```python
from build123d import *

# Parameters (mm, degrees)
SKETCH1_R             = 150.5
BOSS_EXTRUDE1_DEPTH   = 6.35
SKETCH3_R             = 2.6
CUT_EXTRUDE2_DEPTH    = 10
M5X0_8_TAPPED_HOLE1_D = 4.2
CUT_EXTRUDE3_DEPTH    = 10


with BuildPart() as part:
    # Sketch1 → Boss-Extrude1 (new body)
    with BuildSketch(Plane(origin=(-388.281715987, 0, -288.185661777), x_dir=(1, 0, 0), z_dir=(0, 1, 0))):
        Polygon((1747.570833697, -13084.824581071), (1672.514355591, -13084.824581071), (1454.703489965, -13462.084066777), (1492.231729019, -13527.084883536), (1927.853460271, -13527.084883536), (1965.381699324, -13462.084066777), align=None)
        with Locations(Location((1710.042594644, -13357.997843795, 0), (0, 0, 270))):
            Circle(SKETCH1_R, mode=Mode.SUBTRACT)
        with BuildLine():
            Line((1730.692592416, -13114.874577827), (1730.692592416, -13095.074579966))
            ThreePointArc((1730.692592416, -13095.074579966), (1730.472922526, -13094.544249938), (1729.942592497, -13094.324580043))
            Line((1729.942592497, -13094.324580043), (1690.142596792, -13094.324580043))
            ThreePointArc((1690.142596792, -13094.324580043), (1689.612266761, -13094.544249935), (1689.392596873, -13095.074579966))
            Line((1689.392596873, -13095.074579966), (1689.392596873, -13114.874577827))
            ThreePointArc((1689.392596873, -13114.874577827), (1689.612266763, -13115.404907856), (1690.142596792, -13115.62457775))
            Line((1690.142596792, -13115.62457775), (1729.942592497, -13115.62457775))
            ThreePointArc((1729.942592497, -13115.62457775), (1730.472922528, -13115.404907859), (1730.692592416, -13114.874577827))
        make_face(mode=Mode.SUBTRACT)
        with BuildLine():
            Line((1492.669367808, -13507.342898369), (1509.816668952, -13497.442899438))
            ThreePointArc((1509.816668952, -13497.442899438), (1510.166113284, -13496.987494718), (1510.091187977, -13496.418380495))
            Line((1510.091187977, -13496.418380495), (1490.191190123, -13461.950573141))
            ThreePointArc((1490.191190123, -13461.950573141), (1489.735785404, -13461.60112881), (1489.166671181, -13461.676054117))
            Line((1489.166671181, -13461.676054117), (1472.019370034, -13471.57605305))
            ThreePointArc((1472.019370034, -13471.57605305), (1471.669925699, -13472.031457773), (1471.744851013, -13472.600571998))
            Line((1471.744851013, -13472.600571998), (1491.644848864, -13507.068379347))
            ThreePointArc((1491.644848864, -13507.068379347), (1492.100253585, -13507.41782368), (1492.669367808, -13507.342898369))
        make_face(mode=Mode.SUBTRACT)
        with BuildLine():
            Line((1948.065819252, -13471.576053055), (1930.918518105, -13461.676054122))
            ThreePointArc((1930.918518105, -13461.676054122), (1930.349403886, -13461.601128813), (1929.893999164, -13461.95057314))
            Line((1929.893999164, -13461.95057314), (1909.99400131, -13496.418380494))
            ThreePointArc((1909.99400131, -13496.418380494), (1909.919076, -13496.98749472), (1910.268520339, -13497.442899434))
            Line((1910.268520339, -13497.442899434), (1927.415821483, -13507.342898365))
            ThreePointArc((1927.415821483, -13507.342898365), (1927.984935702, -13507.417823673), (1928.440340423, -13507.068379346))
            Line((1928.440340423, -13507.068379346), (1948.340338275, -13472.600571997))
            ThreePointArc((1948.340338275, -13472.600571997), (1948.415263583, -13472.031457775), (1948.065819252, -13471.576053055))
        make_face(mode=Mode.SUBTRACT)
    extrude(amount=BOSS_EXTRUDE1_DEPTH)

    # Sketch3 → Cut-Extrude2 (cut)
    with BuildSketch(Plane(origin=(0, 6.35, 0), x_dir=(1, 0, 0), z_dir=(0, 1, 0))):
        with Locations(Location((1183.987460829, -12990.268662147, 0), (0, 0, 270))):
            Circle(SKETCH3_R)
        with Locations(Location((1146.487460829, -13055.220567431, 0), (0, 0, 270))):
            Circle(SKETCH3_R)
        with Locations(Location((1108.987460829, -13120.172472715, 0), (0, 0, 270))):
            Circle(SKETCH3_R)
        with Locations(Location((1221.487460829, -12925.316756863, 0), (0, 0, 270))):
            Circle(SKETCH3_R)
        with Locations(Location((1258.987460829, -12860.364851579, 0), (0, 0, 270))):
            Circle(SKETCH3_R)
        with Locations(Location((1459.534296487, -12990.268662148, 0), (0, 0, 270))):
            Circle(SKETCH3_R)
        with Locations(Location((1497.034296487, -13055.220567432, 0), (0, 0, 270))):
            Circle(SKETCH3_R)
        with Locations(Location((1534.534296487, -13120.172472716, 0), (0, 0, 270))):
            Circle(SKETCH3_R)
        with Locations(Location((1422.034296487, -12925.316756864, 0), (0, 0, 270))):
            Circle(SKETCH3_R)
        with Locations(Location((1384.534296487, -12860.364851581, 0), (0, 0, 270))):
            Circle(SKETCH3_R)
        with Locations(Location((1321.760878657, -13228.899221759, 0), (0, 0, 270))):
            Circle(SKETCH3_R)
        with Locations(Location((1246.760878657, -13228.899221759, 0), (0, 0, 270))):
            Circle(SKETCH3_R)
        with Locations(Location((1171.760878657, -13228.899221759, 0), (0, 0, 270))):
            Circle(SKETCH3_R)
        with Locations(Location((1396.760878657, -13228.899221759, 0), (0, 0, 270))):
            Circle(SKETCH3_R)
        with Locations(Location((1471.760878657, -13228.899221759, 0), (0, 0, 270))):
            Circle(SKETCH3_R)
    extrude(amount=-CUT_EXTRUDE2_DEPTH, mode=Mode.SUBTRACT)

    # M5x0.8 Tapped Hole1 (through all)
    with Locations(Plane(origin=(0, 6.35, 0), x_dir=(1, 0, 0), z_dir=(0, 1, 0))):
        with Locations((1321.760878658, -12912.312182018), (1321.760878658, -13069.812182018), (1382.033519255, -12924.301155648), (1261.48823806, -12924.301155648), (1185.361877562, -13148.562182018), (1165.608312991, -13090.370057293), (1225.880953589, -13194.765333114), (1417.640803726, -13194.765333114), (1458.159879754, -13148.562182018), (1477.913444324, -13090.370057293)):
            Hole(M5X0_8_TAPPED_HOLE1_D / 2)

    # Sketch9 → Cut-Extrude3 (cut)
    with BuildSketch(Plane(origin=(0, 6.35, 0), x_dir=(1, 0, 0), z_dir=(0, 1, 0))):
        with BuildLine():
            Line((1522.758854804, -13174.820007204), (1515.224433791, -13170.470007204))
            ThreePointArc((1515.224433791, -13170.470007204), (1513.706795701, -13170.270206359), (1512.492382983, -13171.202058012))
            Line((1512.492382983, -13171.202058012), (1504.492382983, -13185.058464472))
            ThreePointArc((1504.492382983, -13185.058464472), (1504.292582138, -13186.576102563), (1505.224433791, -13187.79051528))
            Line((1505.224433791, -13187.79051528), (1512.758854804, -13192.14051528))
            ThreePointArc((1512.758854804, -13192.14051528), (1514.276492894, -13192.340316125), (1515.490905611, -13191.408464472))
            Line((1515.490905611, -13191.408464472), (1523.490905611, -13177.552058012))
            ThreePointArc((1523.490905611, -13177.552058012), (1523.690706456, -13176.034419922), (1522.758854804, -13174.820007204))
        make_face()
        with BuildLine():
            Line((1312.201334792, -12843.238915973), (1312.201334792, -12851.938915973))
            ThreePointArc((1312.201334792, -12851.938915973), (1312.787121229, -12853.353129536), (1314.201334792, -12853.938915973))
            Line((1314.201334792, -12853.938915973), (1330.201334792, -12853.938915973))
            ThreePointArc((1330.201334792, -12853.938915973), (1331.615548354, -12853.353129536), (1332.201334792, -12851.938915973))
            Line((1332.201334792, -12851.938915973), (1332.201334792, -12843.238915973))
            ThreePointArc((1332.201334792, -12843.238915973), (1331.615548354, -12841.824702411), (1330.201334792, -12841.238915973))
            Line((1330.201334792, -12841.238915973), (1314.201334792, -12841.238915973))
            ThreePointArc((1314.201334792, -12841.238915973), (1312.787121229, -12841.824702411), (1312.201334792, -12843.238915973))
        make_face()
        with BuildLine():
            Line((1130.322446377, -13191.377622877), (1137.85686739, -13187.027622877))
            ThreePointArc((1137.85686739, -13187.027622877), (1138.788719043, -13185.81321016), (1138.588918198, -13184.29557207))
            Line((1138.588918198, -13184.29557207), (1130.588918198, -13170.439165609))
            ThreePointArc((1130.588918198, -13170.439165609), (1129.37450548, -13169.507313956), (1127.85686739, -13169.707114801))
            Line((1127.85686739, -13169.707114801), (1120.322446377, -13174.057114801))
            ThreePointArc((1120.322446377, -13174.057114801), (1119.390594725, -13175.271527519), (1119.59039557, -13176.789165609))
            Line((1119.59039557, -13176.789165609), (1127.59039557, -13190.64557207))
            ThreePointArc((1127.59039557, -13190.64557207), (1128.804808287, -13191.577423722), (1130.322446377, -13191.377622877))
        make_face()
    extrude(amount=-CUT_EXTRUDE3_DEPTH, mode=Mode.SUBTRACT)


solid = part.part
```
Build history of the part. All positions in model axes, mm. A direction names the side the tool comes from. Give positions to 0.01 mm unless a question says otherwise; leave off trailing zeros. Loops run counter-clockwise (first coordinate to the right, second up) from the corner with the lowest first, then second, coordinate; pieces in that order, holes last.
Item 1: Slice it at A-A, the plane x = 1198.5. List the corners of the cut face in (y, z), and give its area (3 significant figures).
Answers follow:
outline: (0, 12945.13) - (6.35, 12945.13) - (6.35, 12983.46) - (0, 12983.46) - close; (0, 13156.17) - (6.35, 13156.17) - (6.35, 13238.9) - (0, 13238.9) - close
area: 769 mm2
Item 2: Which spindle directions (+Z, -Z, +X, -X, +Y, -Y) get a long thin tool onto all of the face, cutting with end or side? Do faces 1 (the face through (1549.97, 3.13, 13201.89)), 2 (the face through (1188, 6.35, 13000)). Say none if no direction does.
Answers follow:
face 1: +Y, -Y
face 2: +Z, -Z, +X, -X, +Y
Item 3: Drill centre lines: line 1 (X direction, y = 2.25, z = 13179); line 2 (X direction, y = 5, z = 13207); line 3 (Z direction, x = 1312, y = 1.25). Where is each one in solid material? Low to high.
Answers follow:
line 1: x = 1069.37 to 1091.34, 1104.93 to 1120.87, 1135.53 to 1218.18, 1425.34 to 1507.99, 1522.65 to 1538.59, 1552.18 to 1574.15
line 2: x = 1085.53 to 1096.5, 1121.1 to 1259.88, 1383.65 to 1522.42, 1547.02 to 1557.99
line 3: z = 12796.64 to 12806.14, 12827.44 to 12919.63, 13220 to 13238.9
Item 4: Slice it at C-C, the plane y = 4. Give the number of separate pieces and of enclosed holes in the cut face, and give its area (3 significant figures).
Answers follow:
separate pieces: 1
enclosed holes: 31
area: 66,300 mm2
Item 5: Slice it at D-D, the plane z = 12880. List the corners of the cut face in (x, y).
Answers follow:
outline: (1236.1, 0) - (1407.42, 0) - (1407.42, 6.35) - (1236.1, 6.35) - close
Item 6: Slice it at B-B, the plane z = 12944.5. List the corners of the cut face in (x, y) (3 decimals), and give its area (3 significant figures).
Answers follow:
outline: (1198.865, 0) - (1238.412, 0) - (1238.412, 6.35) - (1198.865, 6.35) - close; (1405.11, 0) - (1444.657, 0) - (1444.657, 6.35) - (1405.11, 6.35) - close
area: 502 mm2
Item 7: Flat gauge pins, fed straight in: pin 1 (2 mm diameter, centred on x = 1187, y = 5, fed in from -Z); pin 2 (1 mm diameter, centred on y = 4, z = 12977.5, fed in from +X); pin 3 (3 mm diameter, centred on y = 2.5, z = 13015.5, fed in from -X). Where does each tip first touch, or does it go through?
Answers follow:
pin 1: stops at z = 12963.32
pin 2: stops at x = 1464
pin 3: stops at x = 1157.01
Item 8: Pull direction X, two halves, no side cores. Call faces 3 (the face through (1176.85, 3.13, 12982.63)), 4 (the face through (1264.118, 3.131, 13208.836)), 5 (the face through (1469.72, 3.13, 12987.91)), 6 (the face through (1112, 3.13, 13191.24)): released by +X, released by -X, zero draft, split by the parting line, or undercut.
Answers follow:
face 3: released by -X
face 4: undercut
face 5: released by +X
face 6: undercut
